The model under review builds one solid part; all positions refer to its coordinate system, in mm. Round coordinates to 2 decimals unless told otherwise and drop trailing zeros. Order: outer loops, then holes, each group sorted by start corner. A loop starts at its lowest first (then second) coordinate and runs counter-clockwise, first axis right, second up.
from build123d import *

# Parameters (mm, degrees)
BOSS_EXTRUDE1_DEPTH                             = 6.35
SKETCH2_W                                       = 149.3748
SKETCH2_H                                       = 287.7714167
CUT_EXTRUDE1_DEPTH                              = 7.35
FILLET1_R                                       = 3
CSK_FOR_10_FLAT_HEAD_MACHINE_SCREW2_D           = 5.1054
CSK_FOR_10_FLAT_HEAD_MACHINE_SCREW2_CSINK_D     = 9.779
CSK_FOR_10_FLAT_HEAD_MACHINE_SCREW2_CSINK_ANGLE = 82
CSK_FOR_10_FLAT_HEAD_MACHINE_SCREW1_D           = 5.1054
CSK_FOR_10_FLAT_HEAD_MACHINE_SCREW1_CSINK_D     = 9.779
CSK_FOR_10_FLAT_HEAD_MACHINE_SCREW1_CSINK_ANGLE = 82
CSK_FOR_10_FLAT_HEAD_MACHINE_SCREW3_D           = 5.1054
CSK_FOR_10_FLAT_HEAD_MACHINE_SCREW3_CSINK_D     = 9.779
CSK_FOR_10_FLAT_HEAD_MACHINE_SCREW3_CSINK_ANGLE = 82
CSK_FOR_10_FLAT_HEAD_MACHINE_SCREW5_D           = 4.9784
CSK_FOR_10_FLAT_HEAD_MACHINE_SCREW5_CSINK_D     = 9.779
CSK_FOR_10_FLAT_HEAD_MACHINE_SCREW5_CSINK_ANGLE = 82
F_5_16_CLEARANCE_HOLE1_D                        = 8.72998
FILLET2_R                                       = 5.5


with BuildPart() as part:
    # Sketch1 → Boss-Extrude1 (new body)
    with BuildSketch(Plane.XY):
        with BuildLine():
            Line((32.5, 94.5), (32.5, 258))
            Line((32.5, 258), (-375.6002, 258))
            Line((-375.6002, 258), (-375.6002, -258))
            Line((-375.6002, -258), (-34.5, -258))
            Line((-34.5, -258), (-34.5, -27.308423609))
            ThreePointArc((-34.5, -27.308423609), (-43.951223006, -2.071230621), (-36.915254237, 23.942932247))
            ThreePointArc((-36.915254237, 23.942932247), (-35.11648189, 27.849193214), (-34.5, 32.105295513))
            Line((-34.5, 32.105295513), (-34.5, 56.5))
            ThreePointArc((-34.5, 56.5), (-28.642135624, 70.642135624), (-14.5, 76.5))
            Line((-14.5, 76.5), (14.5, 76.5))
            ThreePointArc((14.5, 76.5), (27.227922061, 81.772077939), (32.5, 94.5))
        make_face()
    extrude(amount=BOSS_EXTRUDE1_DEPTH)

    # Sketch2 → Cut-Extrude1 (cut, through all)
    with BuildSketch(Plane(origin=(0, 0, 0), x_dir=(-1, 0, 0), z_dir=(0, 0, -1))):
        with Locations((140.2876, 0)):
            Rectangle(SKETCH2_W, SKETCH2_H)
    extrude(amount=-CUT_EXTRUDE1_DEPTH, mode=Mode.SUBTRACT)

    # Fillet1
    fillet1_edges = [part.edges().sort_by_distance(p)[0] for p in [
        (-65.6002, -143.88570835, 3.175),
        (-65.6002, 143.88570835, 3.175),
        (-214.975, 143.88570835, 3.175),
        (-214.975, -143.88570835, 3.175),
    ]]
    fillet(fillet1_edges, radius=FILLET1_R)

    # CSK for #10 Flat Head Machine Screw2 (through all)
    with Locations(Plane.XY.offset(6.35)):
        with Locations((-271, 249.5), (-299, 249.5), (-271, -249.5), (-299, -249.5), (-336, -249.5), (-364, -249.5), (-336, 249.5), (-364, 249.5), (-46, -249.5), (-74, -249.5), (-46, 249.5), (-74, 249.5)):
            CounterSinkHole(CSK_FOR_10_FLAT_HEAD_MACHINE_SCREW2_D / 2, CSK_FOR_10_FLAT_HEAD_MACHINE_SCREW2_CSINK_D / 2, counter_sink_angle=CSK_FOR_10_FLAT_HEAD_MACHINE_SCREW2_CSINK_ANGLE)

    # CSK for #10 Flat Head Machine Screw1 (through all)
    with Locations(Plane.XY.offset(6.35)):
        with Locations((-369.2375, 105.78570835), (-369.2375, 25.27849165), (-369.2375, -25.27849165), (-369.2375, -105.78570835), (-59.2375, 105.78570835), (-59.2375, 0), (-59.2375, -105.78570835)):
            CounterSinkHole(CSK_FOR_10_FLAT_HEAD_MACHINE_SCREW1_D / 2, CSK_FOR_10_FLAT_HEAD_MACHINE_SCREW1_CSINK_D / 2, counter_sink_angle=CSK_FOR_10_FLAT_HEAD_MACHINE_SCREW1_CSINK_ANGLE)

    # CSK for #10 Flat Head Machine Screw3 (through all)
    with Locations(Plane.XY.offset(6.35)):
        with Locations((-227, 17), (-320, 0), (-227, -35), (-227, -17), (-227, 35)):
            CounterSinkHole(CSK_FOR_10_FLAT_HEAD_MACHINE_SCREW3_D / 2, CSK_FOR_10_FLAT_HEAD_MACHINE_SCREW3_CSINK_D / 2, counter_sink_angle=CSK_FOR_10_FLAT_HEAD_MACHINE_SCREW3_CSINK_ANGLE)

    # CSK for #10 Flat Head Machine Screw5 (through all)
    with Locations(Plane.XY.offset(6.35)):
        with Locations((-228.6375, 243), (-187.3625, 243), (-187.3625, -243), (-228.6375, -243)):
            CounterSinkHole(CSK_FOR_10_FLAT_HEAD_MACHINE_SCREW5_D / 2, CSK_FOR_10_FLAT_HEAD_MACHINE_SCREW5_CSINK_D / 2, counter_sink_angle=CSK_FOR_10_FLAT_HEAD_MACHINE_SCREW5_CSINK_ANGLE)

    # 5/16 Clearance Hole1 (through all)
    with Locations(Plane.XY.offset(6.35)):
        with Locations((-208, 243), (-208, -243)):
            Hole(F_5_16_CLEARANCE_HOLE1_D / 2)

    # Fillet2
    fillet2_edges = [part.edges().sort_by_distance(p)[0] for p in [
        (-34.5, -258, 3.175),
        (-375.6002, -258, 3.175),
        (-375.6002, 258, 3.175),
        (32.5, 258, 3.175),
    ]]
    fillet(fillet2_edges, radius=FILLET2_R)


solid = part.part
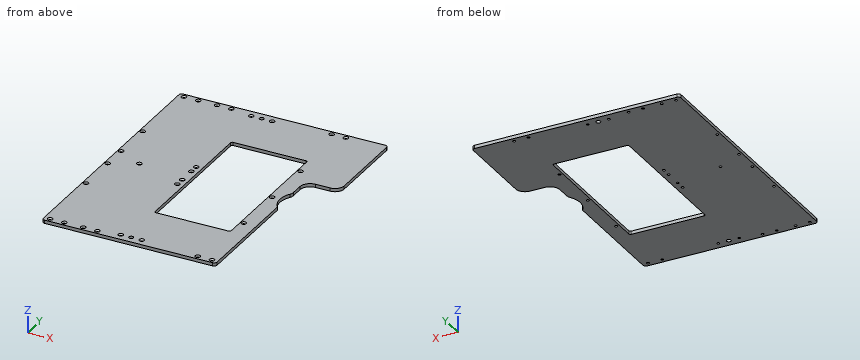
(1) We need section B-B (y = -180.5). Give the boundary of the cut face in (x, z).
(2) To check wall thickness, follow L1, parallel to Y at x = -208, z = 5.25 (3 decimals); L2, parallel to X at y = -127.5, z = 2.25 (3 decimals); L3, parallel to Y at x = -149.5, z = 6. State the ranges of each line that lie inside material, in increasing order.
(3) We need section A-A (x = -154). Give the boundary of the cut face in (y, z).
(4) Clearance check with flat-ended pins moving along their axes: P1, Ø8, axis at x = -271, y = 249.5, coming from the +Z side; P2, Ø1.5, axis at y = -50.5, z = 5, coming from the +X side; P3, Ø1.9, axis at x = 4, z = 2, coming from the -Y side. State where each tip first meets the part, or that it passes through.
Verdict:
1. outline: (-375.6, 0) - (-34.5, 0) - (-34.5, 6.35) - (-375.6, 6.35) - close
2. L1: y = -258 to -247.365, -238.635 to -143.886, 143.886 to 238.635, 247.365 to 258
2. L2: x = -375.6 to -214.975, -65.6 to -34.5
2. L3: y = -258 to -143.89, 143.89 to 258
3. outline: (-258, 0) - (-143.89, 0) - (-143.89, 6.35) - (-258, 6.35) - close; (143.89, 0) - (258, 0) - (258, 6.35) - (143.89, 6.35) - close
4. P1: stops at z = 5.33
4. P2: stops at x = -34.5
4. P3: stops at y = 76.5
